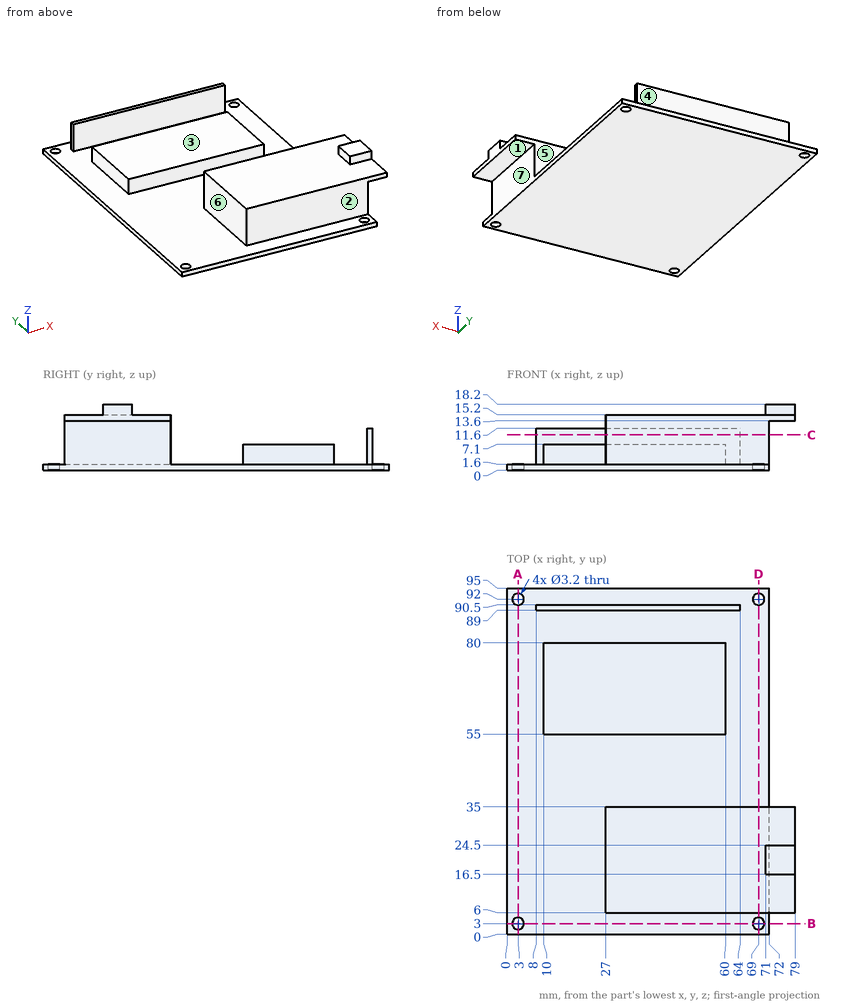
For this review, use the dimensioned drawing (mm, ordinates from the lowest corner) and the shaded views. A direction names the side the tool comes from. Give positions to 0.01 mm unless a question says otherwise; leave off trailing zeros. Order: outer loops, then holes, each group sorted by start corner. A loop starts at its lowest first (then second) coordinate and runs counter-clockwise, first axis right, second up. Notation, with made-up numbers: (-13, 16.5) - (30, 16.5) arc R9 cw to (30, 31.5) - close; hole circle Ø1 at (46, 5.5). An arc over 180 degrees is marked (long way). Use a Markdown table: item, result. Add a question column.
(1) Machinability: for the marked faces 5, 6 and 7, which of the approach directions +Z, -Z, +X, -X, +Y, -Y give a long, thin tool a straight path to every point of the face, cutting with its end or side? Answer none if there is none.
(2) Clearance check with flat-ended pins moving along their axes: P1, Ø3.5, axis at x = 75.5, z = 16, coming from the -Y side; P2, Ø0.9, axis at y = 18.5, z = 17.5, coming from the -X side; P3, Ø2, axis at x = 61.5, z = 6, coming from the +Y side. State where each tip first meets the part, or that it passes through.
(3) Add section C-C on z = 9.75. Give the boundary of the cut face in (x, y), then the cut area to 3 significant figures.
(4) Mouldability with a two-part tool opening along Y and no side actions: class the marked faces 1, 2, 3 and 4 as +Y half, -Y half, draft (parallel to the pull), parting line (faces both ways), or undercut.
(5) Add section D-D on x = 69. Give the boundary of the cut face in (y, z).
(6) Add section B-B on y = 3. Give the boundary of the cut face in (x, z), then the cut area to 3 significant figures.
(7) Wall thickness on probe 1 along X at (y, z) = (92, 0.4); probe 2 along Y at (x, z) = (69, 0.7); probe 3 along Z at (x, y) = (7.5, 31): over which ranges is each line inside the solid? List them lowest first. Write a range as [from, to].
(8) Add section A-A on x = 3. Give the boundary of the cut face in (y, z).
Report:
| question | item | result |
|---|---|---|
| 1 | face 5 | +Z, +X, -X |
| 1 | face 6 | +Z, -X, -Y |
| 1 | face 7 | -Z, +X, +Y, -Y |
| 2 | P1 | stops at y = 6 |
| 2 | P2 | stops at x = 71 |
| 2 | P3 | stops at y = 90.5 |
| 3 | outline | (8, 89) - (64, 89) - (64, 90.5) - (8, 90.5) - close; (27, 6) - (72, 6) - (72, 35) - (27, 35) - close |
| 3 | area | 1,390 mm² |
| 4 | face 1 | draft |
| 4 | face 2 | -Y half |
| 4 | face 3 | undercut |
| 4 | face 4 | +Y half |
| 5 | outline | (0, 0) - (1.4, 0) - (1.4, 1.6) - (0, 1.6) - close; (4.6, 0) - (90.4, 0) - (90.4, 1.6) - (35, 1.6) - (35, 15.2) - (6, 15.2) - (6, 1.6) - (4.6, 1.6) - close; (93.6, 0) - (95, 0) - (95, 1.6) - (93.6, 1.6) - close |
| 6 | outline | (0, 0) - (1.4, 0) - (1.4, 1.6) - (0, 1.6) - close; (4.6, 0) - (67.4, 0) - (67.4, 1.6) - (4.6, 1.6) - close; (70.6, 0) - (72, 0) - (72, 1.6) - (70.6, 1.6) - close |
| 6 | area | 105 mm² |
| 7 | probe 1 | x = [0, 1.4], [4.6, 67.4], [70.6, 72] |
| 7 | probe 2 | y = [0, 1.4], [4.6, 90.4], [93.6, 95] |
| 7 | probe 3 | z = [0, 1.6] |
| 8 | outline | (0, 0) - (1.4, 0) - (1.4, 1.6) - (0, 1.6) - close; (4.6, 0) - (90.4, 0) - (90.4, 1.6) - (4.6, 1.6) - close; (93.6, 0) - (95, 0) - (95, 1.6) - (93.6, 1.6) - close |
